```python
from build123d import *

# Parameters (mm, degrees)
F2_SIZE = 1
F3_R    = 0.5


# Not quite as in the source:
# - a feature names something its author has since deleted; it is built from what else it names


with BuildPart() as f1:
    # F0 (on Front) → F1 (revolve)
    with BuildSketch(Plane.XZ):
        Polygon((-19.8, 15.4426406871), (-19.8, 0), (-16.8, 0), (-16.8, 14.2), (-1, 30), (-1.5, 33), (-1.5, 37), (-3.5, 37), (-3.5, 31.7426406871), (-16.8, 18.4426406871), (-30, 18.4426406871), (-30, 15.4426406871), align=None)
    revolve(axis=Axis((0, 0, 35), (0, 0, 1)))

    # F2
    f2_edges = [f1.edges().sort_by_distance(p)[0] for p in [
        (30, 0, 18.442641),
        (30, 0, 15.442641),
        (19.8, 0, 0),
        (16.8, 0, 0),
    ]]
    chamfer(f2_edges, length=F2_SIZE)

    # F3
    f3_edges = [f1.edges().sort_by_distance(p)[0] for p in [
        (1.5, 0, 37),
        (3.5, 0, 37),
    ]]
    fillet(f3_edges, radius=F3_R)


solid = f1.part
```
Design review of the part built by this model. Coordinates are the model's own, in mm. A direction names the side the tool comes from. Give positions to 0.01 mm unless a question says otherwise; leave off trailing zeros. Loops run counter-clockwise (first coordinate to the right, second up) from the corner with the lowest first, then second, coordinate; pieces in that order, holes last. Notation, with made-up numbers: M 51.25,49.25 L 70.25,49.25 A28 cw 70.25,74.25 Z; hole C 30,41 d7. An arc over 180 degrees is marked long. Return JSON: item names as keys, results as strings. Group by question number.
Item 1: Insertion check: pin 1 Ø17.5 at (x, y) = (-12, 5) entering from +Z; pin 2 Ø4 at (x, z) = (-4, 16) entering from +Y; pin 3 Ø3 at (x, z) = (-9, 6.5) entering from +Y. Each pin has a flat end and moves straight along its axis. Give the tip position at first contact, or say it passes through.
Item 2: Tool access review of faces 4 (the cylindrical face through (1.5, -0.07, 34.77)), 5 (the cylindrical face through (-16.024, -5.046, 7.692)), 6 (the flat face through (-7, 17, 0)): name each direction out of +Z, -Z, +X, -X, +Y, -Y from which nothing blocks a thin tool from reaching the whole face with its end or side.
Item 3: For probe 1 along Y at (x, z) = (0, 6); probe 2 along X at (y, z) = (0, 34), list the stretches that pass through material, from the lowest coordinate up.
Item 4: Mouldability with a two-part tool opening along X and no side actions: class faces 1 (the conical face through (-1.143, -0.36, 31.188)), 2 (the cylindrical face through (-18.9, -5.9, 8.1)), 3 (the flat face through (12, 12, 18.443)) as released by +X, released by -X, zero draft, split by the parting line, or undercut.
Item 5: We need section B-B (z = 27). Give the boundary of the cut face in (x, y), and give its area (3 significant figures).
Item 6: We need section A-A (z = 34.5). Give the boundary of the cut face in (x, y).
Output:
{
 "1": {"pin 1": "stops at z = 30.99", "pin 2": "stops at y = 29.93", "pin 3": "stops at y = 18.32"},
 "2": {"face 4": "+Z", "face 5": "-Z", "face 6": "-Z, +X, -X, +Y, -Y"},
 "3": {"probe 1": "y = -19.8 to -16.8, 16.8 to 19.8", "probe 2": "x = -3.5 to -1.5, 1.5 to 3.5"},
 "4": {"face 1": "undercut", "face 2": "split by the parting line", "face 3": "zero draft"},
 "5": {"outline": "C 0,0 d16.49; hole C 0,0 d8", "area": "163 mm^2"},
 "6": {"outline": "C 0,0 d7; hole C 0,0 d3"}
}
